Design review of the part built by this model. Coordinates are the model's own, in mm. A direction names the side the tool comes from. Coordinates: 2 decimals unless noted, no trailing zeros. Write each loop counter-clockwise with the first axis right and the second up, starting at its lowest first coordinate (ties: lowest second). Pieces come first, ordered by that corner, then holes. Notation, with made-up numbers: (-31, 80) - (-23, 80) arc R19 ccw to (-23, 106) - close; hole circle Ø2 at (-20, 61.25). An arc over 180 degrees is marked (long way). Use a Markdown table: item, result.
from build123d import *

# Parameters (mm, degrees)
F1_R     = 25.4
F2_DEPTH = 5.08
F3_DEPTH = 25.4


with BuildPart() as f2:
    # F1 (on face) → F2 (new body)
    with BuildSketch(Plane.XZ):
        Circle(F1_R)
    extrude(amount=F2_DEPTH)

    # F0 (on Front) → F3 (cut)
    with BuildSketch(Plane.XZ):
        with BuildLine():
            Line((-18.9649743836, -11.5879407846), (-18.6743181879, 12.0507454217))
            ThreePointArc((-18.6743181879, 12.0507454217), (-22.2233201325, 0.2732531593), (-18.9649743836, -11.5879407846))
        make_face()
        with BuildLine():
            Line((-12.2440231208, 18.5481676404), (-12.2440231208, 18.542))
            Line((-12.2440231208, 18.542), (-12.3461767338, 10.2339809879))
            Line((-12.3461767338, 10.2339809879), (-6.35, 18.542))
            Line((-6.35, 18.542), (-3.9468095651, 21.8717470554))
            ThreePointArc((-3.9468095651, 21.8717470554), (-8.2642187046, 20.6313672403), (-12.2440231208, 18.5481676404))
        make_face()
        with BuildLine():
            Line((2.3905855561, 22.0960567907), (0, 18.542))
            Line((0, 18.542), (-11.534660226, 1.393549738))
            Line((-11.534660226, 1.393549738), (0, -18.542))
            Line((0, -18.542), (2.0748165247, -22.1279407399))
            ThreePointArc((2.0748165247, -22.1279407399), (7.4446563645, -20.9410533788), (12.3586706752, -18.4719756426))
            ThreePointArc((12.3586706752, -18.4719756426), (-3.2744047046, -0.079723759), (11.4450647322, 19.0515384753))
            ThreePointArc((11.4450647322, 19.0515384753), (7.0833309726, 21.0660164087), (2.3905855561, 22.0960567907))
        make_face()
        with BuildLine():
            Line((-12.5719566873, -8.1284057478), (-12.6963058315, -18.2415581361))
            ThreePointArc((-12.6963058315, -18.2415581361), (-8.7364017757, -20.4358975583), (-4.4139898466, -21.782270741))
            Line((-4.4139898466, -21.782270741), (-6.35, -18.542))
            Line((-6.35, -18.542), (-12.5719566873, -8.1284057478))
        make_face()
        with BuildLine():
            ThreePointArc((5.688669798, 10.580847501), (2.8540606181, -5.7704887525), (17.2740589748, -13.9841879112))
            ThreePointArc((17.2740589748, -13.9841879112), (22.2186031718, 0.533196112), (16.5833831495, 14.7966897756))
            ThreePointArc((16.5833831495, 14.7966897756), (10.6903796192, 13.8404233779), (5.688669798, 10.580847501))
        make_face()
    extrude(amount=F3_DEPTH, mode=Mode.SUBTRACT)


solid = f2.part
(1) Take a section at A-A on z = 6.5. Write out the cut boundary in (x, y), and give its area (3 significant figures).
Determined:
| item | result |
|---|---|
| outline | (-24.55, -5.08) - (-21.25, -5.08) - (-21.25, 0) - (-24.55, 0) - close; (-18.74, -5.08) - (-8.1, -5.08) - (-8.1, 0) - (-18.74, 0) - close; (-2.28, -5.08) - (2.83, -5.08) - (2.83, 0) - (-2.28, 0) - close; (21.25, -5.08) - (24.55, -5.08) - (24.55, 0) - (21.25, 0) - close |
| area | 114 mm2 |
(2) For L1, parallel to X at y = -2.35, z = -17; L2, parallel to X at y = -0.8, z = 6.5; L3, parallel to X at y = -2.75, z = -8, list the stretches that pass through material, from the lowest coordinate up. Write a range as from..to.
Determined:
| item | result |
|---|---|
| L1 | -18.87..-12.68, -7.27..-0.89, 7.79..18.87 |
| L2 | -24.55..-21.25, -18.74..-8.1, -2.28..2.83, 21.25..24.55 |
| L3 | -24.11..-20.74, -18.92..-6.1, -1.35..4.16, 20.74..24.11 |
(3) Take a section at B-B on x = -9. Write out the cut boundary in (y, z), and give its area (3 significant figures).
Determined:
| item | result |
|---|---|
| outline | (-5.08, -23.75) - (0, -23.75) - (0, -20.32) - (-5.08, -20.32) - close; (-5.08, -14.11) - (0, -14.11) - (0, -2.99) - (-5.08, -2.99) - close; (-5.08, 5.16) - (0, 5.16) - (0, 14.87) - (-5.08, 14.87) - close; (-5.08, 20.32) - (0, 20.32) - (0, 23.75) - (-5.08, 23.75) - close |
| area | 141 mm2 |
(4) Draft analysis for pull direction X (two halves, no side actions). For faces 1 (the flat face through (-8.436, -2.504, -15.051)), 2 (the cylindrical face through (-5.506, -2.504, -24.796)), 3 (the flat face through (0, -5.08, 0)), state which applies: +X half, -X half, draft (parallel to the pull), parting line (faces both ways), or undercut.
Determined:
| item | result |
|---|---|
| face 1 | undercut |
| face 2 | parting line |
| face 3 | draft |
(5) Machinability: for faces 4 (the flat face through (0, 0, 0)), 5 (the cylindrical face through (2.75, -2.504, -5.546)), which of the approach directions +Z, -Z, +X, -X, +Y, -Y give a long, thin tool a straight path to every point of the face, cutting with its end or side? Answer none if there is none.
Determined:
| item | result |
|---|---|
| face 4 | +Z, -Z, +X, -X, +Y |
| face 5 | +Y, -Y |
(6) For pin 1 (3 mm diameter, centred on x = 12.5, y = -3.5, fed in from +Z); pin 2 (3 mm diameter, centred on y = -2.5, z = 11.5, fed in from -X); pin 3 (1.5 mm diameter, centred on y = -4.5, z = 1.5, fed in from -X), all flat-tipped, find the tip position at first contact; note any pin that passes through.
Determined:
| item | result |
|---|---|
| pin 1 | z = 22.89 |
| pin 2 | x = -23.35 |
| pin 3 | x = -25.39 |
